Can you work these out from the drawing? Everything is in mm from the part's minimum corner. A direction names the side the tool comes from. Round coordinates to 2 decimals unless told otherwise and drop trailing zeros. Loops run counter-clockwise (first coordinate to the right, second up) from the corner with the lowest first, then second, coordinate; pieces in that order, holes last. Notation, with made-up numbers: (63.25, 41.5) -> (121.25, 41.5) arc R14 cw to (121.25, 67.5) -> close; hole circle Ø7 at (-32, 23). An arc over 180 degrees is marked (long way). One line per item, written item: value.
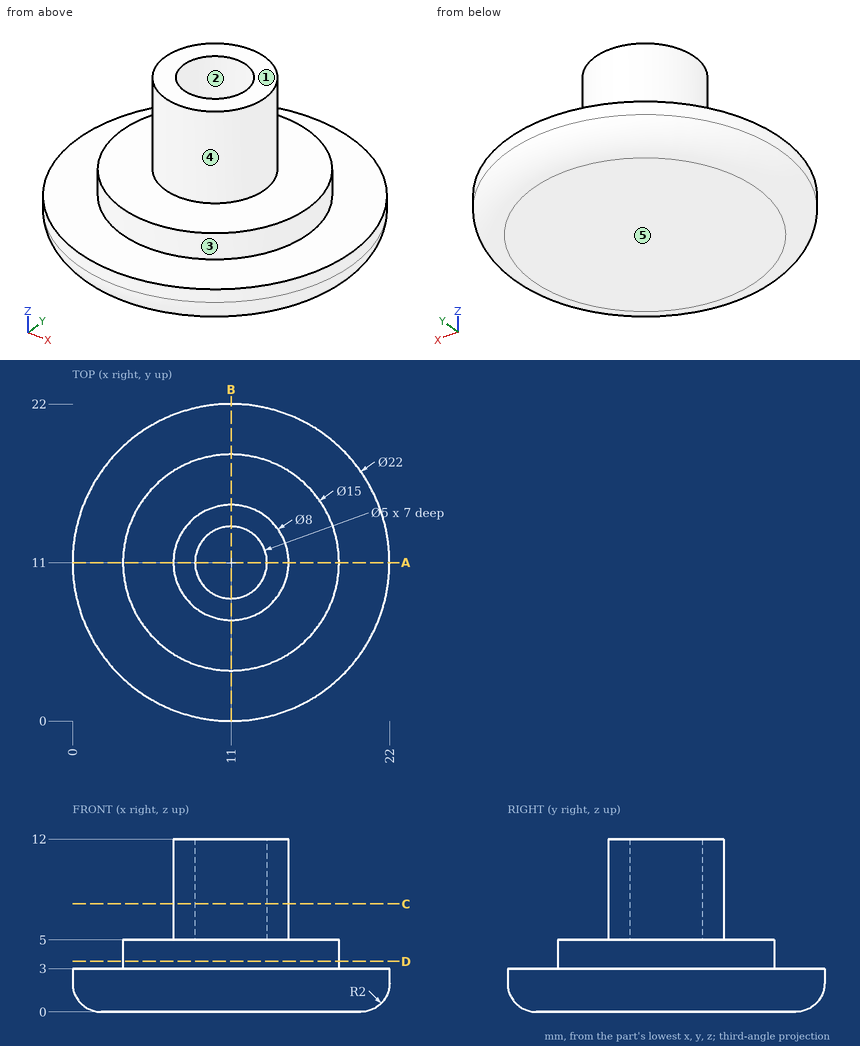
(1) For pin 1 Ø4 at (y, z) = (9.5, 9) entering from +X; pin 2 Ø2.5 at (x, y) = (10.5, 12) entering from +Z, each with a flat end and sliding along its axis, tell me the tip position at first contact or that it passes through.
Results below:
pin 1: stops at x = 15
pin 2: stops at z = 5
(2) Imagine slicing it at D-D on z = 3.5. Write out the boundary of the cut face in (x, y), then the cut area to 3 significant figures.
Results below:
outline: circle Ø15 at (11, 11)
area: 177 mm²
(3) On a 3-axis mill with a long thin cutter (end or side, diameter ignored), from which of +Z, -Z, +X, -X, +Y, -Y can I reach the whole of each face in a straight line? I mean the marked faces 4 and 5. Say none if no direction works.
Results below:
face 4: +Z
face 5: -Z, +X, -X, +Y, -Y
(4) Please list where these lines run through material, in increasing order: L1, parallel to Y at x = 11, z = 7.5; L2, parallel to Z at x = 18.75, y = 13; L3, parallel to Z at x = 10.5, y = 10.
Results below:
L1: y = 7 to 8.5, 13.5 to 15
L2: z = 0 to 3
L3: z = 0 to 5
(5) We'd pull the mould along X, two halves only. Please class the marked faces 1, 2 and 3: +X half, -X half, draft (parallel to the pull), parting line (faces both ways), or undercut.
Results below:
face 1: draft
face 2: undercut
face 3: parting line
(6) Imagine slicing it at A-A on y = 11. Write out the boundary of the cut face in (x, z).
Results below:
outline: (0, 2) arc R2 ccw to (2, 0) -> (20, 0) arc R2 ccw to (22, 2) -> (22, 3) -> (18.5, 3) -> (18.5, 5) -> (15, 5) -> (15, 12) -> (13.5, 12) -> (13.5, 5) -> (8.5, 5) -> (8.5, 12) -> (7, 12) -> (7, 5) -> (3.5, 5) -> (3.5, 3) -> (0, 3) -> close
(7) Imagine slicing it at C-C on z = 7.5. Write out the boundary of the cut face in (x, y), then the cut area to 3 significant figures.
Results below:
outline: circle Ø8 at (11, 11); hole circle Ø5 at (11, 11)
area: 30.6 mm²
